Autodesk Inventor part; units mm, degrees
ref_plane "YZ Plane" through (0, 0, 0) normal (1, 0, 0) x (0, 1, 0)
ref_plane "XZ Plane" through (0, 0, 0) normal (0, 1, 0) x (-1, 0, 0)
ref_plane "XY Plane" through (0, 0, 0) normal (0, 0, 1) x (1, 0, 0)
sketch "Sketch1" plane through (0, 0, 0) normal (1, 0, 0) x (0, 1, 0)
  line L0 (0, 0) -> (15, 0)
  line L1 (15, 0) -> (15, 5)
  line L2 (15, 5) -> (0, 5)
  line L3 (0, 5) -> (0, 0)
  line L4 (10, 5) -> (15, 0)
  dimension "d0" = 15
  dimension "d1" = 5
  dimension "d2" = 5
extrude "Extrusion1" add sketch "Sketch1" along normal blind 90 and the other way blind 5 contours L3 L2 L4 L0
sketch "Sketch2" plane through (-5, 0, 5) normal (0, 0, 1) x (1, 0, 0)
  arc A0 (0, 10) -> (0, -10) centre (0, 0) ccw construction
  arc A1 (-9.7813, 2.08) -> (-9.7813, -2.08) centre (0, 0) ccw construction
  arc A2 (-15.2728, 0.745) -> (-15.2761, -0.675) centre (0, 0) ccw construction
  arc A3 (-15.2761, -0.675) -> (-9.7813, -2.08) centre (-9.8343, 9.1599) ccw construction
  arc A4 (-9.7813, 2.08) -> (-15.2728, 0.745) centre (-9.9572, -9.1586) ccw construction
  line L0 (0, 10) -> (4.16, 10)
  line L1 (0, 10) -> (95, 10)
  line L2 (1.37, 15.291) -> (2.79, 15.291)
  arc A5 (1.37, 15.291) -> (0, 10) centre (11.2397, 9.9126) ccw
  arc A6 (4.16, 10) -> (2.79, 15.291) centre (-7.0797, 9.9126) ccw
  point P0 (5, 0)
  point P1 (2.08, 10)
  dimension "d7" = 4.16
  dimension "d8" = 2.08
  dimension "d9" = 0.745
  dimension "d10" = 1.42
  dimension "d12" = 11.24
  dimension "d13" = 11.24
  dimension "d14" = 5.291
  dimension "d15" = 4.16
  dimension "d16" = 4.16
  dimension "d17" = 1.42
  dimension "d18" = 0.71
  dimension "d19" = 5.291
  dimension "d20" = 11.24
  dimension "d21" = 11.24
sketch "Sketch3" plane through (90, 15, 0) normal (0, 0, -1) x (-1, 0, 0)
  arc A0 (0, 1.075) -> (0, -1.075) centre (0, 0) ccw
  arc A1 (-14.714, 2.915) -> (-14.714, -2.915) centre (0, 0) ccw
  arc A2 (-21.0975, 0.975) -> (-21.0975, -0.975) centre (0, 0) ccw
  arc A3 (-21.0975, -0.975) -> (-14.714, -2.915) centre (-14.5146, 9.2134) ccw
  arc A4 (-14.714, 2.915) -> (-21.0975, 0.975) centre (-14.5146, -9.2134) ccw
  arc A5 (0, 1.075) -> (0, -1.075) centre (0, 0) ccw
  arc A6 (-14.714, 2.915) -> (-14.714, -2.915) centre (0, 0) ccw
  arc A7 (-21.0975, 0.975) -> (-21.0975, -0.975) centre (0, 0) ccw
  arc A8 (-21.0975, -0.975) -> (-14.714, -2.915) centre (-14.5146, 9.2134) ccw
  arc A9 (-14.714, 2.915) -> (-21.0975, 0.975) centre (-14.5146, -9.2134) ccw
  line L0 (0, 0) -> (95, 0)
  line L1 (95, 0) -> (89.17, 0)
  line L2 (91.11, 6.12) -> (93.06, 6.12)
  arc A10 (91.11, 6.12) -> (89.17, 0) centre (101.2907, -0.4747) ccw
  arc A11 (95, 0) -> (93.06, 6.12) centre (82.8793, -0.4747) ccw
  point P0 (90, -15)
  point P1 (0, -15)
  point P2 (0, -15)
  point P3 (92.085, 0)
  dimension "d22" = 2.915
  dimension "d23" = 5.83
  dimension "d24" = 0.975
  dimension "d25" = 1.95
  dimension "d26" = 21.12
  dimension "d27" = 12.13
  dimension "d28" = 12.13
  dimension "d29" = 2.915
  dimension "d30" = 5.83
  dimension "d31" = 0.975
  dimension "d32" = 1.95
  dimension "d33" = 21.12
  dimension "d34" = 12.13
  dimension "d35" = 12.13
  dimension "d36" = 5.83
  dimension "d37" = 5.83
  dimension "d38" = 1.95
  dimension "d39" = 0.975
  dimension "d40" = 6.12
  dimension "d41" = 6.12
  dimension "d42" = 12.13
  dimension "d43" = 12.13
loft "Loft1" add profiles "Sketch2", "Sketch3" contours all / A10 L2 A11 L0
pattern_linear "Rectangular Pattern1" count 11 spacing 8.91 along (1, 0, 0) of "Loft1"
properties part number "lockPin"
Geometry: final body of the model. Coordinates: model frame, mm. A direction names the side the tool comes from. Round coordinates to 2 decimals unless told otherwise and drop trailing zeros. Loops run counter-clockwise (first coordinate to the right, second up) from the corner with the lowest first, then second, coordinate; pieces in that order, holes last. Notation, with made-up numbers: M -39.75,1 L -30.75,1 A15 ccw -30.75,18 Z; hole C 76.5,-29.75 d4. An arc over 180 degrees is marked long. Put each result on its own line as item: value. Start each with the question number.
(1) Material intervals for line 1 along Y through (x, z) = (75, 2.1); line 2 along Z through (x, y) = (60, 19.75); line 3 along Y through (x, z) = (1.5, 3.9), sorted ascending. Write a range as [from, to].
(2) Section query A-A (x = 2). Return loops of the section in (y, z).
(3) Draft query along X for faces 4 (the face through (90, 6, 3)), 5 (the face through (20, 12, 3)), 6 (the face through (43, 8, 0)). Return one class per face: +X half, -X half, draft (parallel to the pull), parting line (faces both ways), or undercut.
(4) Set-up query: faces 1 (the face through (2, 12, 3)), 2 (the face through (89.3, 11.9, 3.1)), 3 (the face through (43, 6, 5)). Return all of +Z, -Z, +X, -X, +Y, -Y with unobstructed straight access to the full face (end or side cutting, diameter ignored); none if empty.
(5) Contact query for flat-ended pins moving along their axis: pin 1 Ø1 at (y, z) = (15.5, 2) entering from +X; pin 2 Ø1 at (x, y) = (42.5, 17) entering from +Z. Output: stop coordinate, or through.
Findings below:
1. line 1: y = [0, 12.9]
1. line 2: z = [0, 1.18]
1. line 3: y = [0, 11.1]
2. outline: M 0,0 L 15,0 L 10,5 L 0,5 Z
3. face 4: +X half
3. face 5: undercut
3. face 6: draft
4. face 1: +Z, +Y
4. face 2: +Z, +X, +Y
4. face 3: +Z, +X, -X, +Y, -Y
5. pin 1: stops at x = 89.21
5. pin 2: stops at z = 3.96
